For this review, take the finished solid that the model builds, in its own axes (mm). A direction names the side the tool comes from. Coordinates: 2 decimals unless noted, no trailing zeros. Loops run counter-clockwise (first coordinate to the right, second up) from the corner with the lowest first, then second, coordinate; pieces in that order, holes last. Notation, with made-up numbers: M 12.25,55 L 39.25,55 A16 ccw 39.25,82 Z; hole C 52,57 d7. An arc over 180 degrees is marked long. Answer as a JSON object with one key per item and string values. Group by question number.
Item 1: Wall thickness on L1, parallel to Y at x = 81, z = 24; L2, parallel to X at y = 145.5, z = 11.5; L3, parallel to Y at x = 182.5, z = 28.5: over which ranges is each line inside the solid? List them lowest first. Write a range as from..to.
Item 2: Add section B-B (x = 160). State the section outline as (y, z) points.
Item 3: Mouldability with a two-part tool opening along Y and no side actions: class faces 1 (the face through (4.283, -2.175, 31.059)), 2 (the face through (193, 104, 6.8)), 3 (the face through (195.276, 81, 31)) as +Y half, -Y half, draft (parallel to the pull), parting line (faces both ways), or undercut.
Item 4: Tool access review of faces 4 (the face through (193, 104, 4.4)), 5 (the face through (3, 133.973, 5)), 6 (the face through (191.276, 80, 30)), 7 (the face through (193, 136.273, 6)), 8 (the face through (190.27, 159.12, 61.48)): name each direction out of +Z, -Z, +X, -X, +Y, -Y from which nothing blocks a thin tool from reaching the whole face with its end or side.
Item 5: Add section A-A (y = 46.5). State the section outline as (x, z) points.
Item 6: Add section C-C (z = 53.5). Count the separate pieces of the cut face and the enclosed holes in it, then the cut area to 3 significant figures.
Item 7: Insertion check: pin 1 (4.5 mm diameter, centred on x = 193.5, z = 6, fed in from -Y); pin 2 (2.5 mm diameter, centred on x = 193, z = 5.5, fed in from -Y); pin 3 (2 mm diameter, centred on x = 193, y = 105, fed in from -Z); pin 4 (3 mm diameter, centred on x = 3.5, y = 126, fed in from -Z). Each pin has a flat end and moves straight along its axis. Give the tip position at first contact, or say it passes through.
Autodesk Inventor part; units mm, degrees
ref_plane "YZ Plane" through (0, 0, 0) normal (1, 0, 0) x (0, 1, 0)
ref_plane "XZ Plane" through (0, 0, 0) normal (0, 1, 0) x (-1, 0, 0)
ref_plane "XY Plane" through (0, 0, 0) normal (0, 0, 1) x (1, 0, 0)
sketch "Sketch1" plane through (0, 0, 0) normal (0, 0, 1) x (1, 0, 0)
  line L0 (13.2756, 161.973) -> (183.2756, 161.973)
  line L1 (193.2756, 151.973) -> (193.2756, 6.973)
  line L2 (183.2756, -3.027) -> (13.2756, -3.027)
  line L3 (3.2756, 6.973) -> (3.2756, 151.973)
  arc A0 (13.2756, 161.973) -> (3.2756, 151.973) centre (13.2756, 151.973) ccw
  arc A1 (193.2756, 151.973) -> (183.2756, 161.973) centre (183.2756, 151.973) ccw
  arc A2 (183.2756, -3.027) -> (193.2756, 6.973) centre (183.2756, 6.973) ccw
  arc A3 (3.2756, 6.973) -> (13.2756, -3.027) centre (13.2756, 6.973) ccw
  circle A4 centre (13.2756, 151.973) radius 1.5
  circle A5 centre (183.2756, 151.973) radius 1.5
  circle A6 centre (183.2756, 6.973) radius 1.5
  circle A7 centre (13.2756, 6.973) radius 1.5
  line L4 (15.2756, 159.973) -> (181.2756, 159.973)
  line L5 (191.2756, 149.973) -> (191.2756, 8.973)
  line L6 (181.2756, -1.027) -> (15.2756, -1.027)
  line L7 (5.2756, 8.973) -> (5.2756, 149.973)
  line L8 (11.2756, 163.973) -> (185.2756, 163.973)
  line L9 (195.2756, 153.973) -> (195.2756, 4.973)
  line L10 (185.2756, -5.027) -> (11.2756, -5.027)
  line L11 (1.2756, 4.973) -> (1.2756, 153.973)
  arc A8 (195.2756, 153.973) -> (185.2756, 163.973) centre (185.2756, 153.973) ccw
  arc A9 (11.2756, 163.973) -> (1.2756, 153.973) centre (11.2756, 153.973) ccw
  arc A10 (1.2756, 4.973) -> (11.2756, -5.027) centre (11.2756, 4.973) ccw
  arc A11 (185.2756, -5.027) -> (195.2756, 4.973) centre (185.2756, 4.973) ccw
  arc A12 (9.8418, 149.9214) -> (16.7094, 154.0246) centre (13.2756, 151.973) ccw
  line L12 (16.7094, 154.0246) -> (13.2761, 159.771)
  line L13 (16.7094, 154.0246) -> (9.8418, 149.9214) construction
  line L14 (9.8418, 149.9214) -> (6.7189, 155.1482)
  arc A13 (15.2756, 159.973) -> (13.2761, 159.771) centre (15.2756, 149.973) ccw
  arc A14 (6.7189, 155.1482) -> (5.2756, 149.973) centre (15.2756, 149.973) ccw
  arc A15 (181.4201, 155.5166) -> (185.7337, 148.8174) centre (183.2756, 151.973) ccw
  arc A16 (185.2426, 10.4559) -> (181.3086, 3.49) centre (183.2756, 6.973) ccw
  arc A17 (16.2722, 4.3233) -> (9.8626, 9.059) centre (13.2756, 6.973) ccw
  line L15 (185.7337, 148.8174) -> (190.8637, 152.8135)
  line L16 (185.7337, 148.8174) -> (181.4201, 155.5166) construction
  line L17 (181.4201, 155.5166) -> (186.7789, 158.3225)
  arc A18 (191.2756, 149.973) -> (190.8637, 152.8135) centre (181.2756, 149.973) ccw
  arc A19 (186.7789, 158.3225) -> (181.2756, 159.973) centre (181.2756, 149.973) ccw
  line L18 (16.2722, 4.3233) -> (12.0222, -0.483)
  line L19 (16.2722, 4.3233) -> (9.8626, 9.059) construction
  line L20 (9.8626, 9.059) -> (6.6833, 3.8571)
  arc A20 (5.2756, 8.973) -> (6.6833, 3.8571) centre (15.2756, 8.973) ccw
  arc A21 (12.0222, -0.483) -> (15.2756, -1.027) centre (15.2756, 8.973) ccw
  line L21 (185.2426, 10.4559) -> (191.1069, 7.144)
  line L22 (185.2426, 10.4559) -> (181.3086, 3.49) construction
  line L23 (181.3086, 3.49) -> (186.5944, 0.5048)
  arc A22 (181.2756, -1.027) -> (186.5944, 0.5048) centre (181.2756, 8.973) ccw
  arc A23 (191.1069, 7.144) -> (191.2756, 8.973) centre (181.2756, 8.973) ccw
  point P0 (0, 0)
  point P1 (193.2756, -3.027)
  point P2 (193.2756, 161.973)
  point P3 (3.2756, -3.027)
  point P4 (191.2756, -1.027)
  point P5 (191.2756, 159.973)
  point P6 (5.2756, -1.027)
  point P7 (195.2756, -5.027)
  point P8 (195.2756, 163.973)
  point P9 (1.2756, -5.027)
  dimension "d0" = 190
  dimension "d1" = 165
  dimension "d2" = 10
  dimension "a" = 3
  dimension "d4" = 3
  dimension "d5" = 3
  dimension "d6" = 3
  dimension "d7" = 186
  dimension "d8" = 161
  dimension "d9" = 2
  dimension "d10" = 2
  dimension "d11" = 2
  dimension "d12" = 2
  dimension "d14" = 194
  dimension "d15" = 169
  dimension "d16" = 2
  dimension "d17" = 2
  dimension "d18" = 10
  dimension "d19" = 8
  dimension "d20" = 8
  dimension "d21" = 8
  dimension "d22" = 8
extrude "Extrusion1" add sketch "Sketch1" along normal blind 63 contours L8 A8 L9 A11 L10 A10 L11 A9
extrude "Extrusion2" add sketch "Sketch1" along normal blind 60 contours L0 A1 L1 A2 L2 A3 L3 A0
sketch "Sketch2" plane through (195.2756, 4.973, 0) normal (1, 0, 0) x (0, 0, -1)
  line L0 (0, 0) -> (0, 149) construction
  line L1 (0, 149) -> (-63, 149) construction
  line L2 (-63, 0) -> (-63, 149) construction
  line L3 (0, 0) -> (-63, 0) construction
  line L4 (-11.4, 114.7) -> (0, 114.7)
  line L5 (0, 114.7) -> (0, 131.3)
  line L6 (0, 131.3) -> (-11.4, 131.3)
  line L7 (-11.4, 131.3) -> (-11.4, 114.7)
  line L8 (0, 0) -> (0, 149)
  line L9 (0, 94.8) -> (-6.8, 94.8)
  line L10 (-6.8, 94.8) -> (-6.8, 103.2)
  line L11 (-6.8, 103.2) -> (0, 103.2)
  line L12 (0, 103.2) -> (0, 94.8)
  line L13 (0, 94.8) -> (-4.4, 94.8)
  line L14 (-4.4, 94.8) -> (-4.4, 103.2)
  line L15 (-4.4, 103.2) -> (0, 103.2)
  line L16 (0, 103.2) -> (0, 94.8)
  circle A0 centre (-10, 69.8) radius 3.95
  point P0 (0, -4.973)
  dimension "d27" = 11.4
  dimension "d28" = 16.6
  dimension "d29" = 17.7
  dimension "d30" = 11.5
  dimension "d31" = 6.8
  dimension "d32" = 8.4
  dimension "d33" = 4.4
  dimension "d34" = 7.9
  dimension "d35" = 25
  dimension "d36" = 10
extrude "Extrusion3" cut sketch "Sketch2" against normal blind 10 contours L7 L6 L5 L4 | L14 L9 L10 L11 | A0
sketch "Sketch3" plane through (1.2756, 4.973, 0) normal (-1, 0, 0) x (0, 0, 1)
  line L0 (0, 149) -> (0, 0)
  line L1 (0, 0) -> (63, 0)
  line L2 (63, 149) -> (63, 0)
  line L3 (0, 149) -> (63, 149)
  line L4 (0, 4) -> (0, 145)
  line L5 (0, 129) -> (10.2, 129)
  line L6 (10.2, 129) -> (10.2, 111.5)
  line L7 (10.2, 111.5) -> (0, 111.5)
  line L8 (0, 111.5) -> (0, 129)
  point P0 (0, -4.973)
  point P1 (0, 111.5)
  dimension "d39" = 17.5
  dimension "d40" = 10.2
  dimension "d41" = 20
extrude "Extrusion4" cut sketch "Sketch3" against normal blind 10 contours L5 L6 L7 L0
equation "\"d4\" = a"
equation "\"d5\" = a"
equation "\"d6\" = a"
properties part number "Housing"
From the geometry:
{
 "1": {"L1": "y = -5.03..-1.03, 159.97..163.97", "L2": "x = 1.28..5.28, 191.28..195.28", "L3": "y = -5.03..-0.95, 2.82..5.69, 8.26..10.9, 148.05..150.69, 153.26..156.08, 159.9..163.97"},
 "2": {"outline": "M -5.03,0 L -1.03,0 L -1.03,60 L -3.03,60 L -3.03,63 L -5.03,63 Z; M 159.97,0 L 163.97,0 L 163.97,63 L 161.97,63 L 161.97,60 L 159.97,60 Z"},
 "3": {"face 1": "-Y half", "face 2": "undercut", "face 3": "draft"},
 "4": {"face 4": "+X", "face 5": "-Z, +X, -X", "face 6": "+Z, -Z", "face 7": "-Z, +X", "face 8": "+Z"},
 "5": {"outline": "M 1.28,0 L 5.28,0 L 5.28,60 L 3.28,60 L 3.28,63 L 1.28,63 Z; M 191.28,0 L 195.28,0 L 195.28,63 L 193.28,63 L 193.28,60 L 191.28,60 Z"},
 "6": {"separate pieces": "1", "enclosed holes": "5", "area": "3,130 mm²"},
 "7": {"pin 1": "stops at y = -3.05", "pin 2": "stops at y = -2.65", "pin 3": "stops at z = 0", "pin 4": "stops at z = 10.2"}
}
